Here's how the part is built. I have some questions about the finished solid (model axes, mm). A direction names the side the tool comes from. Give positions to 0.01 mm unless a question says otherwise; leave off trailing zeros. Write each loop counter-clockwise with the first axis right and the second up, starting at its lowest first coordinate (ties: lowest second). Pieces come first, ordered by that corner, then holes. Notation, with made-up numbers: (73.5, 72.25) -> (132.5, 72.25) arc R13 ccw to (132.5, 87.25) -> close; hole circle Ø9 at (-17.5, -29.5). An arc over 180 degrees is marked (long way). Use CSV: the item, a comma, the result in double quotes. Start each with the question number.
(1) Which directions (+Z, -Z, +X, -X, +Y, -Y) give clear straight access to the entire face, cutting with the end or side of a thin tool? Please do faces 1 (the cylindrical face through (35.56, 2.96, 1.52)), 2 (the cylindrical face through (-57.311, 55.374, 1.479)).
(2) Suppose I cut it at D-D on y = 47. List the corners of the cut face in (x, z) for me, plus the area to 3 significant figures.
(3) Suppose I cut it at A-A on x = 12. List the corners of the cut face in (y, z) for me, plus the area to 3 significant figures.
(4) Suppose I cut it at B-B on y = 37.4. List the corners of the cut face in (x, z) for me, plus the area to 4 significant figures.
(5) If we mould it in two halves opening along Y, with no side actions, what happens to faces 3 (the flat face through (-3, 18, 3)), 4 (the cylindrical face through (26.606, 17.598, 1.521)), 5 (the cylindrical face through (52.76, 55.296, 1.479))? For each: pulls with the +Y half, pulls with the -Y half, needs draft (parallel to the pull), parting line crosses it, or undercut.
(6) For pin 1 Ø1 at (x, y) = (-30.5, 11) entering from +Z, with a flat end and sliding along its axis, tell me the tip position at first contact or that it passes through.
(7) Suppose I cut it at C-C on x = -45.5. List the corners of the cut face in (y, z) for me (3 decimals).
(8) I need wall thicknesses on L1, parallel to Y at x = 42, z = 2.1 (3 decimals); L2, parallel to X at y = 27, z = 2.6; L3, parallel to Y at x = 5, z = 2.5. Which ranges of each line are inside material? Lowest first, please. Write a range as [from, to].
from build123d import *

# Parameters (mm, degrees)
EXTRUDE_2_DEPTH     = 3
SKETCH_5_R          = 1.625
CUT_EXTRUDE_3_DEPTH = 3


with BuildPart() as part:
    # 草图1 → 凸台-拉伸2 (new body)
    with BuildSketch(Plane.XY):
        with BuildLine():
            Line((-53.814137931, 0), (49.185862069, 0))
            ThreePointArc((49.185862069, 0), (52.721395975, 1.464466094), (54.185862069, 5))
            Line((54.185862069, 5), (54.185862069, 51.8))
            ThreePointArc((54.185862069, 51.8), (52.721395975, 55.335533906), (49.185862069, 56.8))
            Line((49.185862069, 56.8), (31.685862069, 56.8))
            ThreePointArc((31.685862069, 56.8), (30.271648507, 57.385786438), (29.685862069, 58.8))
            Line((29.685862069, 58.8), (29.685862069, 61.8))
            ThreePointArc((29.685862069, 61.8), (29.100075631, 63.214213562), (27.685862069, 63.8))
            Line((27.685862069, 63.8), (-32.314137931, 63.8))
            ThreePointArc((-32.314137931, 63.8), (-33.728351493, 63.214213562), (-34.314137931, 61.8))
            Line((-34.314137931, 61.8), (-34.314137931, 58.8))
            ThreePointArc((-34.314137931, 58.8), (-34.899924369, 57.385786438), (-36.314137931, 56.8))
            Line((-36.314137931, 56.8), (-53.814137931, 56.8))
            ThreePointArc((-53.814137931, 56.8), (-57.349671837, 55.335533906), (-58.814137931, 51.8))
            Line((-58.814137931, 51.8), (-58.814137931, 5))
            ThreePointArc((-58.814137931, 5), (-57.349671837, 1.464466094), (-53.814137931, 0))
        make_face()
    extrude(amount=EXTRUDE_2_DEPTH)

    # 草图5 → 切除-拉伸3 (cut)
    with BuildSketch(Plane.XY.offset(3)):
        with Locations((-29.684137931, 60.8)):
            Circle(SKETCH_5_R)
        with Locations((25.055862069, 60.8)):
            Circle(SKETCH_5_R)
        with Locations((-29.684137931, 17.11)):
            Circle(SKETCH_5_R)
        with Locations((25.055862069, 17.11)):
            Circle(SKETCH_5_R)
        with Locations((-55.314137931, 15.4)):
            Circle(SKETCH_5_R)
        with Locations((-55.314137931, 41.4)):
            Circle(SKETCH_5_R)
        with Locations((50.685862069, 37.4)):
            Circle(SKETCH_5_R)
        with Locations((50.685862069, 19.4)):
            Circle(SKETCH_5_R)
        with BuildLine():
            Line((-48.906226665, 50.8), (-36.722049198, 50.8))
            ThreePointArc((-36.722049198, 50.8), (-35.019398812, 50.094739119), (-34.314137931, 48.392088734))
            Line((-34.314137931, 48.392088734), (-34.314137931, 15.517911266))
            ThreePointArc((-34.314137931, 15.517911266), (-33.60887705, 13.815260881), (-31.906226665, 13.11))
            Line((-31.906226665, 13.11), (-23.722049198, 13.11))
            ThreePointArc((-23.722049198, 13.11), (-22.019398812, 12.404739119), (-21.314137931, 10.702088734))
            Line((-21.314137931, 10.702088734), (-21.314137931, 8.407911266))
            ThreePointArc((-21.314137931, 8.407911266), (-22.019398812, 6.705260881), (-23.722049198, 6))
            Line((-23.722049198, 6), (-48.906226665, 6))
            ThreePointArc((-48.906226665, 6), (-50.60887705, 6.705260881), (-51.314137931, 8.407911266))
            Line((-51.314137931, 8.407911266), (-51.314137931, 48.392088734))
            ThreePointArc((-51.314137931, 48.392088734), (-50.60887705, 50.094739119), (-48.906226665, 50.8))
        make_face()
        with BuildLine():
            Line((-48.814137931, 4.625), (-41.814137931, 4.625))
            ThreePointArc((-41.814137931, 4.625), (-40.189137931, 3), (-41.814137931, 1.375))
            Line((-41.814137931, 1.375), (-48.814137931, 1.375))
            ThreePointArc((-48.814137931, 1.375), (-50.439137931, 3), (-48.814137931, 4.625))
        make_face()
        with BuildLine():
            Line((37.185862069, 4.625), (44.185862069, 4.625))
            ThreePointArc((44.185862069, 4.625), (45.810862069, 3), (44.185862069, 1.375))
            Line((44.185862069, 1.375), (37.185862069, 1.375))
            ThreePointArc((37.185862069, 1.375), (35.560862069, 3), (37.185862069, 4.625))
        make_face()
        with BuildLine():
            Line((-48.814137931, 55.425), (-41.814137931, 55.425))
            ThreePointArc((-41.814137931, 55.425), (-40.189137931, 53.8), (-41.814137931, 52.175))
            Line((-41.814137931, 52.175), (-48.814137931, 52.175))
            ThreePointArc((-48.814137931, 52.175), (-50.439137931, 53.8), (-48.814137931, 55.425))
        make_face()
        with BuildLine():
            Line((37.185862069, 55.425), (44.185862069, 55.425))
            ThreePointArc((44.185862069, 55.425), (45.810862069, 53.8), (44.185862069, 52.175))
            Line((44.185862069, 52.175), (37.185862069, 52.175))
            ThreePointArc((37.185862069, 52.175), (35.560862069, 53.8), (37.185862069, 55.425))
        make_face()
        with BuildLine():
            Line((29.685862069, 48.392088734), (29.685862069, 15.517911266))
            ThreePointArc((29.685862069, 15.517911266), (28.980601188, 13.815260881), (27.277950802, 13.11))
            Line((27.277950802, 13.11), (19.093773335, 13.11))
            ThreePointArc((19.093773335, 13.11), (17.39112295, 12.404739119), (16.685862069, 10.702088734))
            Line((16.685862069, 10.702088734), (16.685862069, 8.407911266))
            ThreePointArc((16.685862069, 8.407911266), (17.39112295, 6.705260881), (19.093773335, 6))
            Line((19.093773335, 6), (44.277950802, 6))
            ThreePointArc((44.277950802, 6), (45.980601188, 6.705260881), (46.685862069, 8.407911266))
            Line((46.685862069, 8.407911266), (46.685862069, 48.392088734))
            ThreePointArc((46.685862069, 48.392088734), (45.980601188, 50.094739119), (44.277950802, 50.8))
            Line((44.277950802, 50.8), (32.093773335, 50.8))
            ThreePointArc((32.093773335, 50.8), (30.39112295, 50.094739119), (29.685862069, 48.392088734))
        make_face()
        with BuildLine():
            Line((-23.814137931, 54.8), (-23.814137931, 24))
            ThreePointArc((-23.814137931, 24), (-22.935458275, 21.878679656), (-20.814137931, 21))
            Line((-20.814137931, 21), (16.185862069, 21))
            ThreePointArc((16.185862069, 21), (18.307182413, 21.878679656), (19.185862069, 24))
            Line((19.185862069, 24), (19.185862069, 54.8))
            ThreePointArc((19.185862069, 54.8), (18.307182413, 56.921320344), (16.185862069, 57.8))
            Line((16.185862069, 57.8), (-20.814137931, 57.8))
            ThreePointArc((-20.814137931, 57.8), (-22.935458275, 56.921320344), (-23.814137931, 54.8))
        make_face()
    extrude(amount=-CUT_EXTRUDE_3_DEPTH, mode=Mode.SUBTRACT)


solid = part.part
Geometry says:
1,face 1,"+Z, -Z"
1,face 2,"+Z, -Z, -X, +Y"
2,outline,"(-58.81, 0) -> (-51.31, 0) -> (-51.31, 3) -> (-58.81, 3) -> close; (-34.31, 0) -> (-23.81, 0) -> (-23.81, 3) -> (-34.31, 3) -> close; (19.19, 0) -> (29.69, 0) -> (29.69, 3) -> (19.19, 3) -> close; (46.69, 0) -> (54.19, 0) -> (54.19, 3) -> (46.69, 3) -> close"
2,area,"108 mm²"
3,outline,"(0, 0) -> (21, 0) -> (21, 3) -> (0, 3) -> close; (57.8, 0) -> (63.8, 0) -> (63.8, 3) -> (57.8, 3) -> close"
3,area,"81.0 mm²"
4,outline,"(-58.81, 0) -> (-51.31, 0) -> (-51.31, 3) -> (-58.81, 3) -> close; (-34.31, 0) -> (-23.81, 0) -> (-23.81, 3) -> (-34.31, 3) -> close; (19.19, 0) -> (29.69, 0) -> (29.69, 3) -> (19.19, 3) -> close; (46.69, 0) -> (49.06, 0) -> (49.06, 3) -> (46.69, 3) -> close; (52.31, 0) -> (54.19, 0) -> (54.19, 3) -> (52.31, 3) -> close"
4,area,"98.25 mm²"
5,face 3,"needs draft"
5,face 4,"undercut"
5,face 5,"pulls with the +Y half"
6,pin 1,"through"
7,outline,"(0, 0) -> (1.375, 0) -> (1.375, 3) -> (0, 3) -> close; (4.625, 0) -> (6, 0) -> (6, 3) -> (4.625, 3) -> close; (50.8, 0) -> (52.175, 0) -> (52.175, 3) -> (50.8, 3) -> close; (55.425, 0) -> (56.8, 0) -> (56.8, 3) -> (55.425, 3) -> close"
8,L1,"[0, 1.375], [4.625, 6], [50.8, 52.175], [55.425, 56.8]"
8,L2,"[-58.81, -51.31], [-34.31, -23.81], [19.19, 29.69], [46.69, 54.19]"
8,L3,"[0, 21], [57.8, 63.8]"
